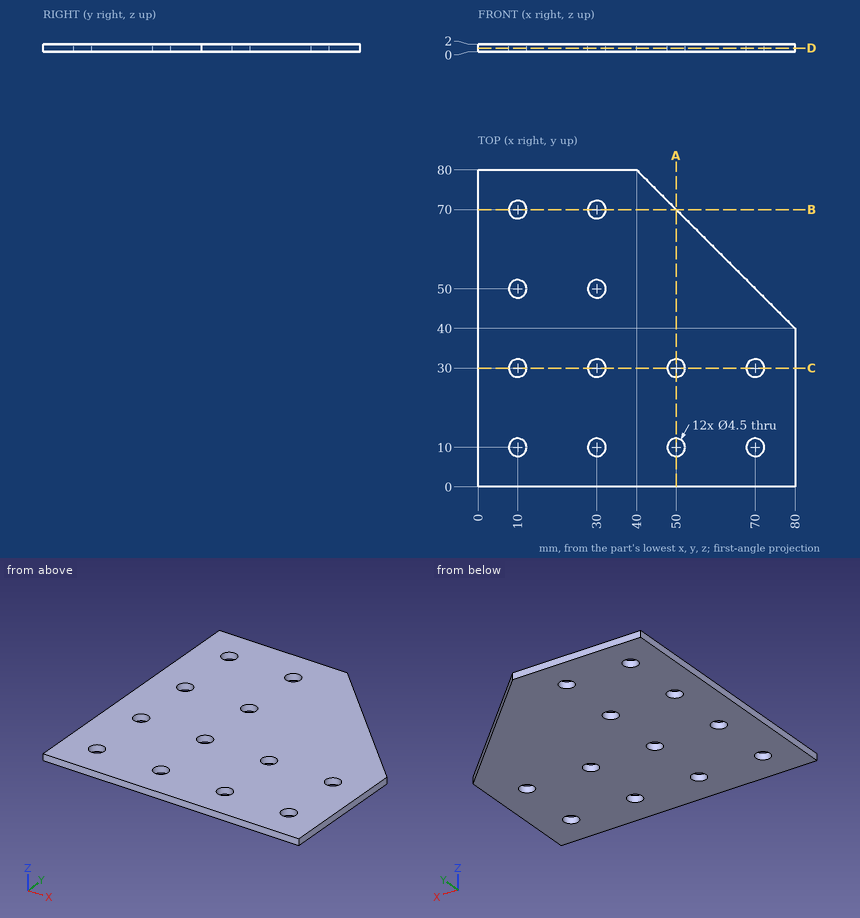
Print and shaded views of the part. All mm, measured from the part's lowest x, y and z. Coordinates: 2 decimals unless noted, no trailing zeros. Write each loop counter-clockwise with the first axis right and the second up, starting at its lowest first coordinate (ties: lowest second). Pieces come first, ordered by that corner, then holes. Notation, with made-up numbers: (-26, 20) - (-2, 20) arc R34 cw to (-2, 50) - close; hole circle Ø3 at (-14.5, 73). An arc over 180 degrees is marked (long way). One line per question, with ' | ' between items. Start each with the question number.
Q1. Cut at B-B, the plane y = 70. List the corners of the cut face in (x, z).
Q2. Pin check, flat tip, straight feed: pin 1 (1 mm diameter, centred on x = 64.5, z = 0.5, fed in from +Y). Stop position of the tip, or through.
Q3. Cut at D-D, the plane z = 0.95. Give the number of separate pieces and of enclosed holes in the cut face, then the cut area to 3 significant figures.
Q4. Cut at A-A, the plane x = 50. List the corners of the cut face in (y, z).
Q5. Drill centre lines: line 1 (Y direction, x = 30, z = 0.7); line 2 (X direction, y = 9, z = 0.1); line 3 (Y direction, x = 70, z = 0.6). Where is each one in solid material? Low to high. Write a range as [from, to].
Q6. Cut at C-C, the plane y = 30. List the corners of the cut face in (x, z).
Answer below:
1) outline: (0, 0) - (7.75, 0) - (7.75, 2) - (0, 2) - close; (12.25, 0) - (27.75, 0) - (27.75, 2) - (12.25, 2) - close; (32.25, 0) - (50, 0) - (50, 2) - (32.25, 2) - close
2) pin 1: y = 56
3) separate pieces: 1 | enclosed holes: 12 | area: 5,410 mm^2
4) outline: (0, 0) - (7.75, 0) - (7.75, 2) - (0, 2) - close; (12.25, 0) - (27.75, 0) - (27.75, 2) - (12.25, 2) - close; (32.25, 0) - (70, 0) - (70, 2) - (32.25, 2) - close
5) line 1: [0, 7.75], [12.25, 27.75], [32.25, 47.75], [52.25, 67.75], [72.25, 80] | line 2: [0, 7.98], [12.02, 27.98], [32.02, 47.98], [52.02, 67.98], [72.02, 80] | line 3: [0, 7.75], [12.25, 27.75], [32.25, 50]
6) outline: (0, 0) - (7.75, 0) - (7.75, 2) - (0, 2) - close; (12.25, 0) - (27.75, 0) - (27.75, 2) - (12.25, 2) - close; (32.25, 0) - (47.75, 0) - (47.75, 2) - (32.25, 2) - close; (52.25, 0) - (67.75, 0) - (67.75, 2) - (52.25, 2) - close; (72.25, 0) - (80, 0) - (80, 2) - (72.25, 2) - close
